```python
from build123d import *

# Parameters (mm, degrees)
BOSS_EXTRUDE1_DEPTH     = 3
FILLET1_R               = 10
SKETCH2_R               = 3
CUT_EXTRUDE1_DEPTH      = 1
CUT_EXTRUDE1_DEPTH_BACK = 4


with BuildPart() as part:
    # Sketch1 → Boss-Extrude1 (new body)
    with BuildSketch(Plane(origin=(0, 0, 0), x_dir=(1, 0, 0), z_dir=(0, 1, 0))):
        with BuildLine():
            Line((-189.549594269, 163.005985511), (-189.549594269, 15))
            Line((-189.549594269, 15), (-189.549594269, -15))
            Line((-189.549594269, -15), (-189.549594269, -163.005985511))
            ThreePointArc((-189.549594269, -163.005985511), (-170.779451396, -182.577049436), (-150, -200))
            Line((-150, -200), (150, -200))
            ThreePointArc((150, -200), (170.779451396, -182.577049436), (189.549594269, -163.005985511))
            Line((189.549594269, -163.005985511), (189.549594269, -15))
            Line((189.549594269, -15), (189.549594269, 15))
            Line((189.549594269, 15), (189.549594269, 163.005985511))
            ThreePointArc((189.549594269, 163.005985511), (0, 250), (-189.549594269, 163.005985511))
        make_face()
        with BuildLine():
            ThreePointArc((-83, -15), (-86.535533906, -13.535533906), (-88, -10))
            Line((-88, -10), (-88, 10))
            ThreePointArc((-88, 10), (-86.535533906, 13.535533906), (-83, 15))
            Line((-83, 15), (-58, 15))
            ThreePointArc((-58, 15), (-54.464466094, 13.535533906), (-53, 10))
            Line((-53, 10), (-53, -10))
            ThreePointArc((-53, -10), (-54.464466094, -13.535533906), (-58, -15))
            Line((-58, -15), (-83, -15))
        make_face(mode=Mode.SUBTRACT)
        with BuildLine():
            Line((53, -10), (53, 10))
            ThreePointArc((53, 10), (54.464466094, 13.535533906), (58, 15))
            Line((58, 15), (83, 15))
            ThreePointArc((83, 15), (86.535533906, 13.535533906), (88, 10))
            Line((88, 10), (88, -10))
            ThreePointArc((88, -10), (86.535533906, -13.535533906), (83, -15))
            Line((83, -15), (58, -15))
            ThreePointArc((58, -15), (54.464466094, -13.535533906), (53, -10))
        make_face(mode=Mode.SUBTRACT)
    extrude(amount=BOSS_EXTRUDE1_DEPTH)

    # Fillet1
    fillet1_edges = [part.edges().sort_by_distance(p)[0] for p in [
        (189.549594269, 1.5, 163.005985511),
        (150, 1.5, 200),
        (-150, 1.5, 200),
        (-189.549594269, 1.5, 163.005985511),
        (-189.549594269, 1.5, -163.005985511),
        (189.549594269, 1.5, -163.005985511),
    ]]
    fillet(fillet1_edges, radius=FILLET1_R)

    # Sketch2 → Cut-Extrude1 (cut, two sides)
    with BuildSketch(Plane.XZ) as cut_extrude1_sk:
        with Locations((-172.549594269, -124.75)):
            Circle(SKETCH2_R)
        with Locations((-172.549594269, -75.25)):
            Circle(SKETCH2_R)
        with Locations((-111.549594269, -124.75)):
            Circle(SKETCH2_R)
        with Locations((-111.549594269, -75.25)):
            Circle(SKETCH2_R)
        with Locations((111.549594269, -75.25)):
            Circle(SKETCH2_R)
        with Locations((172.549594269, -75.25)):
            Circle(SKETCH2_R)
        with Locations((172.549594269, -124.75)):
            Circle(SKETCH2_R)
        with Locations((111.549594269, -124.75)):
            Circle(SKETCH2_R)
        with Locations((172.549594269, 75.25)):
            Circle(SKETCH2_R)
        with Locations((172.549594269, 124.75)):
            Circle(SKETCH2_R)
        with Locations((111.549594269, 124.75)):
            Circle(SKETCH2_R)
        with Locations((111.549594269, 75.25)):
            Circle(SKETCH2_R)
        with Locations((-172.549594269, 75.25)):
            Circle(SKETCH2_R)
        with Locations((-111.549594269, 75.25)):
            Circle(SKETCH2_R)
        with Locations((-111.549594269, 124.75)):
            Circle(SKETCH2_R)
        with Locations((-172.549594269, 124.75)):
            Circle(SKETCH2_R)
        with Locations((-122, 183)):
            Circle(SKETCH2_R)
        with Locations((-72.5, 183)):
            Circle(SKETCH2_R)
        with Locations((72.5, 183)):
            Circle(SKETCH2_R)
        with Locations((122, 183)):
            Circle(SKETCH2_R)
    extrude(amount=CUT_EXTRUDE1_DEPTH, mode=Mode.SUBTRACT)
    extrude(cut_extrude1_sk.sketch, amount=-CUT_EXTRUDE1_DEPTH_BACK, mode=Mode.SUBTRACT)


solid = part.part
```
Geometry: final body of the model. Coordinates: model frame, mm. Give positions to 0.01 mm unless a question says otherwise; leave off trailing zeros. Loops run counter-clockwise (first coordinate to the right, second up) from the corner with the lowest first, then second, coordinate; pieces in that order, holes last. Notation, with made-up numbers: (4.5, 73.25) -> (29.5, 73.25) arc R28 ccw to (29.5, 111.25) -> close; hole circle Ø9 at (33, -19). An arc over 180 degrees is marked (long way). Use CSV: the item, a comma, the result in double quotes.
(1) Ray query, line 1 along X through (y, z) = (2.2, 7); line 2 along Z through (x, y) = (174.5, 1.65); line 3 along Z through (x, y) = (110, 2.7). Return the intervals inside material, ascending. Write a range as [from, to].
From the geometry:
line 1,"[-189.55, -88], [-53, 53], [88, 189.55]"
line 2,"[-179.02, -127.03], [-122.47, -77.53], [-72.97, 72.97], [77.53, 122.47], [127.03, 179.02]"
line 3,"[-224.5, -127.32], [-122.18, -77.82], [-72.68, 72.68], [77.82, 122.18], [127.32, 200]"
(2) First-contact query: P1, Ø5, axis at x = -172.55, z = 75.25, coming from the -Y side; P2, Ø1.5, axis at x = -47.5, y = 1, coming from the -Z side; P3, Ø9.5, axis at x = -111.55, z = -124.75, coming from the +Y side; P4, Ø1.5, axis at x = 67, y = 1.5, coming from the -Z side. Flat tips, straight axial feed; report the tip coordinate or a pass-through.
From the geometry:
P1,"through"
P2,"z = -245.59"
P3,"y = 3"
P4,"z = -241.06"
(3) Cut plane A-A (y = 1.1). Count the separate pieces of the cut face and the enclosed holes in it, plus the area to 3 significant figures.
From the geometry:
separate pieces,"1"
enclosed holes,"22"
area,"157,000 mm^2"
(4) Cut plane B-B (x = 134.5). Output: boundary loops of the cut face in (y, z), plus the area to 3 significant figures.
From the geometry:
outline,"(0, -210.74) -> (3, -210.74) -> (3, 200) -> (0, 200) -> close"
area,"1,230 mm^2"
(5) Cut plane C-C (z = -194). Output: boundary loops of the cut face in (x, y), plus the area to 3 significant figures.
From the geometry:
outline,"(-157.68, 0) -> (157.68, 0) -> (157.68, 3) -> (-157.68, 3) -> close"
area,"946 mm^2"
